```python
from build123d import *

# Parameters (mm, degrees)
SKETCH1_W           = 22.5
SKETCH1_H           = 36.6
BOSS_EXTRUDE1_DEPTH = 18.65
SKETCH1_3_W         = 22.3
SKETCH1_3_H         = 11.7
BOSS_EXTRUDE2_DEPTH = 17.2
SKETCH1_4_W         = 11.8
SKETCH1_4_H         = 3.2
BOSS_EXTRUDE3_DEPTH = 2.6
CUT_EXTRUDE1_REACH  = 44.59
BOSS_EXTRUDE4_DEPTH = 15.8
SKETCH5_R           = 1
BOSS_EXTRUDE5_DEPTH = 1.25
SKETCH6_W           = 5
SKETCH6_H           = 2.5
BOSS_EXTRUDE6_DEPTH = 5
CUT_EXTRUDE2_REACH  = 58.881
SKETCH7_R           = 1.425
SKETCH1_5_R         = 3.725
SKETCH1_5_R_2       = 2.625
BOSS_EXTRUDE7_DEPTH = 0.35
SKETCH1_6_R         = 2.05
BOSS_EXTRUDE8_DEPTH = 1.85
BOSS_EXTRUDE9_DEPTH = 9
CUT_EXTRUDE3_REACH  = 64.008
SKETCH8_R           = 1.5


with BuildPart() as part:
    # Sketch1 → Boss-Extrude1 (new body)
    with BuildSketch(Plane(origin=(0, 0, 0), x_dir=(1, 0, 0), z_dir=(0, 1, 0))):
        with Locations((0, 7.3)):
            Rectangle(SKETCH1_W, SKETCH1_H)
    extrude(amount=-BOSS_EXTRUDE1_DEPTH)

    # Sketch1<3> → Boss-Extrude2 (add)
    with BuildSketch(Plane(origin=(0, 0, 0), x_dir=(1, 0, 0), z_dir=(0, 1, 0))):
        with Locations((0, 31.45)):
            Rectangle(SKETCH1_3_W, SKETCH1_3_H)
    extrude(amount=-BOSS_EXTRUDE2_DEPTH)

    # Sketch1<4> → Boss-Extrude3 (add)
    with BuildSketch(Plane(origin=(0, 0, 0), x_dir=(1, 0, 0), z_dir=(0, 1, 0))):
        with Locations((0, 30.9)):
            Rectangle(SKETCH1_4_W, SKETCH1_4_H)
    boss_extrude3 = extrude(amount=BOSS_EXTRUDE3_DEPTH)

    # Sketch3 → Cut-Extrude1 (cut, up to next)
    with BuildSketch(Plane(origin=(0, 0, -25.6), x_dir=(-1, 0, 0), z_dir=(0, 0, -1)), mode=Mode.PRIVATE) as cut_extrude1_sk1:
        with BuildLine():
            ThreePointArc((11.15, -8.600000119), (10.085885996, -13.353672651), (7.096654141, -17.2))
            Line((7.096654141, -17.2), (11.15, -17.2))
            Line((11.15, -17.2), (11.15, -8.600000119))
        make_face()
    cut_extrude1_tool1 = extrude(cut_extrude1_sk1.sketch, amount=CUT_EXTRUDE1_REACH, mode=Mode.PRIVATE) & part.part
    # Sketch3 → Cut-Extrude1 (cut, up to next)
    with BuildSketch(Plane(origin=(0, 0, -25.6), x_dir=(-1, 0, 0), z_dir=(0, 0, -1)), mode=Mode.PRIVATE) as cut_extrude1_sk2:
        with BuildLine():
            Line((-11.15, -17.2), (-7.096654141, -17.2))
            ThreePointArc((-7.096654141, -17.2), (-10.085886021, -13.353672597), (-11.15, -8.6))
            Line((-11.15, -8.6), (-11.15, -17.2))
        make_face()
    cut_extrude1_tool2 = extrude(cut_extrude1_sk2.sketch, amount=CUT_EXTRUDE1_REACH, mode=Mode.PRIVATE) & part.part
    # Sketch3 → Cut-Extrude1 (cut, up to next)
    with BuildSketch(Plane(origin=(0, 0, -25.6), x_dir=(-1, 0, 0), z_dir=(0, 0, -1)), mode=Mode.PRIVATE) as cut_extrude1_sk3:
        with BuildLine():
            ThreePointArc((7.096654141, 0), (10.085886047, -3.846327457), (11.15, -8.600000119))
            Line((11.15, -8.600000119), (11.15, 0))
            Line((11.15, 0), (7.096654141, 0))
        make_face()
    cut_extrude1_tool3 = extrude(cut_extrude1_sk3.sketch, amount=CUT_EXTRUDE1_REACH, mode=Mode.PRIVATE) & part.part
    # Sketch3 → Cut-Extrude1 (cut, up to next)
    with BuildSketch(Plane(origin=(0, 0, -25.6), x_dir=(-1, 0, 0), z_dir=(0, 0, -1)), mode=Mode.PRIVATE) as cut_extrude1_sk4:
        with BuildLine():
            Line((-11.15, 0), (-11.15, -8.6))
            ThreePointArc((-11.15, -8.6), (-10.085886021, -3.846327403), (-7.096654141, 0))
            Line((-7.096654141, 0), (-11.15, 0))
        make_face()
    cut_extrude1_tool4 = extrude(cut_extrude1_sk4.sketch, amount=CUT_EXTRUDE1_REACH, mode=Mode.PRIVATE) & part.part
    add(cut_extrude1_tool1.solids().sort_by_distance((-9.984236, -15.135971, -25.6))[0], mode=Mode.SUBTRACT)
    add(cut_extrude1_tool2.solids().sort_by_distance((9.984236, -15.135971, -25.6))[0], mode=Mode.SUBTRACT)
    add(cut_extrude1_tool3.solids().sort_by_distance((-9.984236, -2.064029, -25.6))[0], mode=Mode.SUBTRACT)
    add(cut_extrude1_tool4.solids().sort_by_distance((9.984236, -2.064029, -25.6))[0], mode=Mode.SUBTRACT)

    # Sketch4 → Boss-Extrude4 (add)
    with BuildSketch(Plane(origin=(0, 0, -37.3), x_dir=(-1, 0, 0), z_dir=(0, 0, -1))):
        with BuildLine():
            Line((6.651503589, -1.2), (-6.651503589, -1.2))
            ThreePointArc((-6.651503589, -1.2), (-9.95, -8.6), (-6.651503589, -16))
            Line((-6.651503589, -16), (6.651503589, -16))
            ThreePointArc((6.651503589, -16), (9.95, -8.6), (6.651503589, -1.2))
        make_face()
    extrude(amount=BOSS_EXTRUDE4_DEPTH)

    # Sketch5 → Boss-Extrude5 (add)
    with BuildSketch(Plane(origin=(0, 0, -53.1), x_dir=(-1, 0, 0), z_dir=(0, 0, -1))):
        with Locations((0, -8.6)):
            Circle(SKETCH5_R)
    extrude(amount=BOSS_EXTRUDE5_DEPTH)

    # Mirror1: Boss-Extrude3 across plane
    add(boss_extrude3.mirror(Plane.ZX.offset(-8.6)))

    # Sketch6 → Boss-Extrude6 (add)
    with BuildSketch(Plane.XY.offset(11)):
        with Locations((0, -8.6)):
            Rectangle(SKETCH6_W, SKETCH6_H)
    extrude(amount=BOSS_EXTRUDE6_DEPTH)

    # Sketch7 → Cut-Extrude2 (cut, up to next)
    with BuildSketch(Plane(origin=(0, -7.35, 0), x_dir=(1, 0, 0), z_dir=(0, 1, 0)), mode=Mode.PRIVATE) as cut_extrude2_sk1:
        with Locations(Location((0, -13.5, 0), (0, 0, 270))):
            Circle(SKETCH7_R)
    cut_extrude2_tool1 = extrude(cut_extrude2_sk1.sketch, amount=-CUT_EXTRUDE2_REACH, mode=Mode.PRIVATE) & part.part
    add(cut_extrude2_tool1.solids().sort_by_distance((0, -7.35, 13.5))[0], mode=Mode.SUBTRACT)

    # Sketch1<5> → Boss-Extrude7 (add)
    with BuildSketch(Plane(origin=(0, 0, 0), x_dir=(1, 0, 0), z_dir=(0, 1, 0))):
        with Locations(Location((0, 0, 0), (0, 0, 270))):
            Circle(SKETCH1_5_R)
        with Locations(Location((0, 0, 0), (0, 0, 270))):
            Circle(SKETCH1_5_R_2, mode=Mode.SUBTRACT)
    extrude(amount=BOSS_EXTRUDE7_DEPTH)

    # Sketch1<6> → Boss-Extrude8 (add)
    with BuildSketch(Plane(origin=(0, 0, 0), x_dir=(1, 0, 0), z_dir=(0, 1, 0))):
        with Locations(Location((0, 11.075, 0), (0, 0, 270))):
            Circle(SKETCH1_6_R)
    extrude(amount=BOSS_EXTRUDE8_DEPTH)

    # Sketch1<7> → Boss-Extrude9 (add)
    with BuildSketch(Plane(origin=(0, 0, 0), x_dir=(1, 0, 0), z_dir=(0, 1, 0))):
        with BuildLine():
            ThreePointArc((-1.886796226, 1.825), (-2.625, 0), (-1.886796226, -1.825))
            Line((-1.886796226, -1.825), (1.886796226, -1.825))
            ThreePointArc((1.886796226, -1.825), (2.433461022, -0.984323348), (2.625, 0))
            ThreePointArc((2.625, 0), (2.433461022, 0.984323348), (1.886796226, 1.825))
            Line((1.886796226, 1.825), (-1.886796226, 1.825))
        make_face()
    extrude(amount=BOSS_EXTRUDE9_DEPTH)

    # Sketch8 → Cut-Extrude3 (cut, up to next)
    with BuildSketch(Plane.XZ.offset(18.65), mode=Mode.PRIVATE) as cut_extrude3_sk1:
        with Locations(Location((8.65, -20.5, 0), (0, 0, 270))):
            Circle(SKETCH8_R)
    cut_extrude3_tool1 = extrude(cut_extrude3_sk1.sketch, amount=-CUT_EXTRUDE3_REACH, mode=Mode.PRIVATE) & part.part
    # Sketch8 → Cut-Extrude3 (cut, up to next)
    with BuildSketch(Plane.XZ.offset(18.65), mode=Mode.PRIVATE) as cut_extrude3_sk2:
        with Locations(Location((-8.65, -20.5, 0), (0, 0, 270))):
            Circle(SKETCH8_R)
    cut_extrude3_tool2 = extrude(cut_extrude3_sk2.sketch, amount=-CUT_EXTRUDE3_REACH, mode=Mode.PRIVATE) & part.part
    add(cut_extrude3_tool1.solids().sort_by_distance((8.65, -18.65, -20.5))[0], mode=Mode.SUBTRACT)
    add(cut_extrude3_tool2.solids().sort_by_distance((-8.65, -18.65, -20.5))[0], mode=Mode.SUBTRACT)


solid = part.part
```
CAD build for the part. Positions are in the model's coordinates, mm. A direction names the side the tool comes from. Coordinates: 2 decimals unless noted, no trailing zeros. Write each loop counter-clockwise with the first axis right and the second up, starting at its lowest first coordinate (ties: lowest second). Pieces come first, ordered by that corner, then holes.
(1) 3-axis set-ups, long thin cutter, end or side, ignore diameter. For faces 1 (the face through (2.5, -9, 13)), 2 (the face through (0.217, -9.576, -53.716)), 3 (the face through (0, 1, -29.3)), 4 (the face through (0, -18, -29.3)): which of +Z, -Z, +X, -X, +Y, -Y reach the whole face in a straight line?
(2) Cut at D-D, the plane x = -8.65. List the corners of the cut face in (y, z).
(3) Drill centre lines: probe 1 along X at (y, z) = (-11.5, -20.5); probe 2 along Y at (x, z) = (4.5, 4.5); probe 3 along Z at (x, y) = (7, -1.25). Where is each one in solid material? Low to high.
(4) Cut at A-A, the plane z = -20.5. List the corners of the cut face in (x, y).
(5) Two-plate mould, pull along Z, no slides. Class faces 5 (the face through (0, -7, -53.1)), 6 (the face through (0, 2.6, -31)), 7 (the face through (0.62, 0.91, -9.12)): +Z half, -Z half, draft (parallel to the pull), parting line (faces both ways), or undercut.
(6) Cut at B-B, the plane y = 1. List the corners of the cut face in (x, z) (3 decimals).
(7) Cut at C-C, the plane z = 13.5. List the corners of the cut face in (x, y) (3 decimals), and give its area (4 significant figures).
(8) Flat gauge pins, fed straight in: pin 1 (2.5 mm diameter, centred on x = 0.5, z = 13, fed in from -Y); pin 2 (8 mm diameter, centred on x = -3.5, z = -41.5, fed in from -Y); pin 3 (1.3 mm diameter, centred on x = 1, y = -19, fed in from -Z). Where does each tip first touch, or does it go through?
Geometry says:
1. face 1: +Z, +X, +Y, -Y
1. face 2: -Z
1. face 3: +X, -X, +Y
1. face 4: +X, -X, -Y
2. outline: (-18.65, -25.6) - (-15.64, -25.6) - (-15.64, -37.3) - (-13.52, -37.3) - (-13.52, -53.1) - (-3.68, -53.1) - (-3.68, -37.3) - (-1.56, -37.3) - (-1.56, -25.6) - (0, -25.6) - (0, -22) - (-18.65, -22) - close; (-18.65, -19) - (0, -19) - (0, 11) - (-18.65, 11) - close
3. probe 1: x = -11.25 to -10.15, -7.15 to 7.15, 10.15 to 11.25
3. probe 2: y = -18.65 to 0
3. probe 3: z = -37.3 to 11
4. outline: (-11.25, -18.65) - (-10.15, -18.65) - (-10.15, 0) - (-11.25, 0) - close; (-7.15, -18.65) - (7.15, -18.65) - (7.15, 0) - (-7.15, 0) - close; (10.15, -18.65) - (11.25, -18.65) - (11.25, 0) - (10.15, 0) - close
5. face 5: -Z half
5. face 6: draft
5. face 7: undercut
6. outline: (-5.9, -32.5) - (5.9, -32.5) - (5.9, -29.3) - (-5.9, -29.3) - close; circle Ø4.1 at (0, -11.075); (-1.887, -1.825) - (1.887, -1.825) arc R2.625 ccw to (1.887, 1.825) - (-1.887, 1.825) arc R2.625 ccw to start
7. outline: (-2.5, -9.85) - (-1.425, -9.85) - (-1.425, -7.35) - (-2.5, -7.35) - close; (1.425, -9.85) - (2.5, -9.85) - (2.5, -7.35) - (1.425, -7.35) - close
7. area: 5.375 mm2
8. pin 1: stops at y = -9.85
8. pin 2: stops at y = -16
8. pin 3: stops at z = -32.5
